Read the model definition and answer for the solid it produces. Units are mm, in the model's axes. Face numbers are marked on the shaded views. A direction names the side the tool comes from. Round coordinates to 2 decimals unless told otherwise and drop trailing zeros. Order: outer loops, then holes, each group sorted by start corner. A loop starts at its lowest first (then second) coordinate and runs counter-clockwise, first axis right, second up. Notation, with made-up numbers: (85, -8.75) - (107, -8.75) arc R16 ccw to (107, -1.75) - close; hole circle Ø2 at (38.25, -29.75). An arc over 180 degrees is marked (long way). Answer as a JSON object with one key per item and string values. Group by question number.
Q1. A cutting plane is placed at C-C on z = -47.75. Determine the outline of the cut face in (x, y) (3 decimals), and give its area (3 significant figures).
Q2. A tool of negligible diameter and unlimited length cuts with its end or side. For the marked faces 1 and 2, from which of +Z, -Z, +X, -X, +Y, -Y can it reach the whole face along a straight path? Write none if from no direction.
Q3. Given pin 1 Ø2 at (y, z) = (-19.5, -39) entering from +X; pin 2 Ø1 at (y, z) = (-30.5, -42.5) entering from +X; pin 3 Ø5 at (y, z) = (21.5, -49) entering from +X; pin 4 Ø1 at (x, y) = (6.5, -25) entering from +Z, each flat-ended and moving along its own axis, determine where each tip first touches the part or whether it passes through.
Q4. A cutting plane is placed at A-A on x = 12.5. Determine the outline of the cut face in (y, z) (3 decimals), and give its area (3 significant figures).
Q5. A cutting plane is placed at B-B on y = -30.1. Determine the outline of the cut face in (x, z) (3 decimals), and give its area (3 significant figures).
Q6. A cutting plane is placed at D-D on z = -1. Determine the outline of the cut face in (x, y).
Q7. Consider line 1 (Y direction, x = 3.7, z = -47.75) (3 decimals); line 2 (Y direction, x = 10.65, z = 45) (3 decimals); line 3 (Y direction, x = 1.2, z = -61.09). Determine where each line is inside the solid, lowest interval first.
```python
from build123d import *

# Parameters (mm, degrees)
SKETCH1_W            = 133.35
SKETCH1_H            = 76.2
BOSS_EXTRUDE1_DEPTH  = 5
FILLET1_R            = 3.175
SKETCH2_R            = 3.025
CUT_EXTRUDE1_DEPTH   = 77.955608145
SKETCH5_R            = 3.25
SKETCH5_R_2          = 1.665
BOSS_EXTRUDE2_DEPTH  = 2
CUT_EXTRUDE2_START   = -6
SKETCH6_R            = 1.665
CUT_EXTRUDE2_DEPTH   = 6
SKETCH8_R            = 3.75
BOSS_EXTRUDE4_DEPTH  = 9
SKETCH9_R            = 1.665
CUT_EXTRUDE3_DEPTH   = 5
M4_CLEARANCE_HOLE1_D = 4.8
SKETCH16_R           = 4.25
SKETCH16_R_2         = 2.4
CUT_EXTRUDE4_DEPTH   = 2.5


with BuildPart() as part:
    # Sketch1 → Boss-Extrude1 (new body)
    with BuildSketch(Plane(origin=(0, 0, 0), x_dir=(0, 0, -1), z_dir=(1, 0, 0))):
        Rectangle(SKETCH1_W, SKETCH1_H)
    extrude(amount=BOSS_EXTRUDE1_DEPTH)

    # Fillet1
    fillet1_edges = [part.edges().sort_by_distance(p)[0] for p in [
        (2.5, -38.1, -66.675),
        (2.5, -38.1, 66.675),
        (2.5, 38.1, 66.675),
        (2.5, 38.1, -66.675),
    ]]
    fillet(fillet1_edges, radius=FILLET1_R)

    # Sketch2 → Cut-Extrude1 (cut, through all)
    with BuildSketch(Plane.ZY):
        with Locations((-61.09, -22.225)):
            Circle(SKETCH2_R)
        with Locations((-61.09, 22.225)):
            Circle(SKETCH2_R)
        with Locations((61.09, -22.225)):
            Circle(SKETCH2_R)
        with Locations((61.09, 22.225)):
            Circle(SKETCH2_R)
    extrude(amount=-CUT_EXTRUDE1_DEPTH, mode=Mode.SUBTRACT)

    # Sketch5 → Boss-Extrude2 (add)
    # profile 1 of 4: a face of its own
    with BuildSketch(Plane(origin=(5, 0, 0), x_dir=(0, 0, -1), z_dir=(1, 0, 0))):
        with Locations((-52.75, 23)):
            Circle(SKETCH5_R)
        with Locations((-52.75, 23)):
            Circle(SKETCH5_R_2, mode=Mode.SUBTRACT)
    # profile 2 of 4: a face of its own
    with BuildSketch(Plane(origin=(5, 0, 0), x_dir=(0, 0, -1), z_dir=(1, 0, 0))):
        with Locations((-52.75, -12)):
            Circle(SKETCH5_R)
        with Locations((-52.75, -12)):
            Circle(SKETCH5_R_2, mode=Mode.SUBTRACT)
    # profile 3 of 4: a face of its own
    with BuildSketch(Plane(origin=(5, 0, 0), x_dir=(0, 0, -1), z_dir=(1, 0, 0))):
        with Locations((47.75, 23)):
            Circle(SKETCH5_R)
        with Locations((47.75, 23)):
            Circle(SKETCH5_R_2, mode=Mode.SUBTRACT)
    # profile 4 of 4: a face of its own
    with BuildSketch(Plane(origin=(5, 0, 0), x_dir=(0, 0, -1), z_dir=(1, 0, 0))):
        with Locations((47.75, -12)):
            Circle(SKETCH5_R)
    extrude(amount=BOSS_EXTRUDE2_DEPTH)

    # Sketch6 → Cut-Extrude2 (cut)
    with BuildSketch(Plane(origin=(7, 0, 0), x_dir=(0, 0, -1), z_dir=(1, 0, 0)).offset(CUT_EXTRUDE2_START)):
        with Locations((-52.75, -12)):
            Circle(SKETCH6_R)
        with Locations((-52.75, 23)):
            Circle(SKETCH6_R)
        with Locations((47.75, -12)):
            Circle(SKETCH6_R)
        with Locations((47.75, 23)):
            Circle(SKETCH6_R)
    extrude(amount=CUT_EXTRUDE2_DEPTH, mode=Mode.SUBTRACT)

    # Sketch8 → Boss-Extrude4 (add)
    with BuildSketch(Plane(origin=(5, 0, 0), x_dir=(0, 0, -1), z_dir=(1, 0, 0))):
        with Locations((-45, -30.1)):
            Circle(SKETCH8_R)
        with Locations((-45, 30.1)):
            Circle(SKETCH8_R)
        with Locations((42, 30.1)):
            Circle(SKETCH8_R)
        with Locations((42, -30.1)):
            Circle(SKETCH8_R)
    extrude(amount=BOSS_EXTRUDE4_DEPTH)

    # Sketch9 → Cut-Extrude3 (cut)
    with BuildSketch(Plane(origin=(14, 0, 0), x_dir=(0, 0, -1), z_dir=(1, 0, 0))):
        with Locations((-45, -30.1)):
            Circle(SKETCH9_R)
        with Locations((-45, 30.1)):
            Circle(SKETCH9_R)
        with Locations((42, 30.1)):
            Circle(SKETCH9_R)
        with Locations((42, -30.1)):
            Circle(SKETCH9_R)
    extrude(amount=-CUT_EXTRUDE3_DEPTH, mode=Mode.SUBTRACT)

    # M4 Clearance Hole1 (through all)
    with Locations(Plane(origin=(-0.0007, 0, 61.8815), x_dir=(0, 0, -1), z_dir=(-1, 0, 0))):
        with Locations((0, 0), (123.763, 0)):
            Hole(M4_CLEARANCE_HOLE1_D / 2)

    # Sketch16 → Cut-Extrude4 (cut)
    # profile 1 of 6: a face of its own
    with BuildSketch(Plane(origin=(5, 0, 0), x_dir=(0, 0, -1), z_dir=(1, 0, 0))):
        with Locations((-61.8815, 0)):
            Circle(SKETCH16_R)
        with Locations((-61.8815, 0)):
            Circle(SKETCH16_R_2, mode=Mode.SUBTRACT)
    # profile 2 of 6: a face of its own
    with BuildSketch(Plane(origin=(5, 0, 0), x_dir=(0, 0, -1), z_dir=(1, 0, 0))):
        with BuildLine():
            ThreePointArc((-61.8815, -4.25), (-66.1315, 0), (-61.8815, 4.25))
            Line((-61.8815, 4.25), (-66.675, 4.25))
            Line((-66.675, 4.25), (-66.675, -4.25))
            Line((-66.675, -4.25), (-61.8815, -4.25))
        make_face()
    # profile 3 of 6: a face of its own
    with BuildSketch(Plane(origin=(5, 0, 0), x_dir=(0, 0, -1), z_dir=(1, 0, 0))):
        with Locations((-61.8815, 0)):
            Circle(SKETCH16_R_2)
    # profile 4 of 6: a face of its own
    with BuildSketch(Plane(origin=(5, 0, 0), x_dir=(0, 0, -1), z_dir=(1, 0, 0))):
        with Locations((61.8815, 0)):
            Circle(SKETCH16_R)
        with Locations((61.8815, 0)):
            Circle(SKETCH16_R_2, mode=Mode.SUBTRACT)
    # profile 5 of 6: a face of its own
    with BuildSketch(Plane(origin=(5, 0, 0), x_dir=(0, 0, -1), z_dir=(1, 0, 0))):
        with BuildLine():
            Line((66.675, 4.25), (61.8815, 4.25))
            ThreePointArc((61.8815, 4.25), (64.88670382, 3.00520382), (66.1315, 0))
            ThreePointArc((66.1315, 0), (64.88670382, -3.00520382), (61.8815, -4.25))
            Line((61.8815, -4.25), (66.675, -4.25))
            Line((66.675, -4.25), (66.675, 4.25))
        make_face()
    # profile 6 of 6: a face of its own
    with BuildSketch(Plane(origin=(5, 0, 0), x_dir=(0, 0, -1), z_dir=(1, 0, 0))):
        with Locations((61.8815, 0)):
            Circle(SKETCH16_R_2)
    extrude(amount=-CUT_EXTRUDE4_DEPTH, mode=Mode.SUBTRACT)


solid = part.part
```
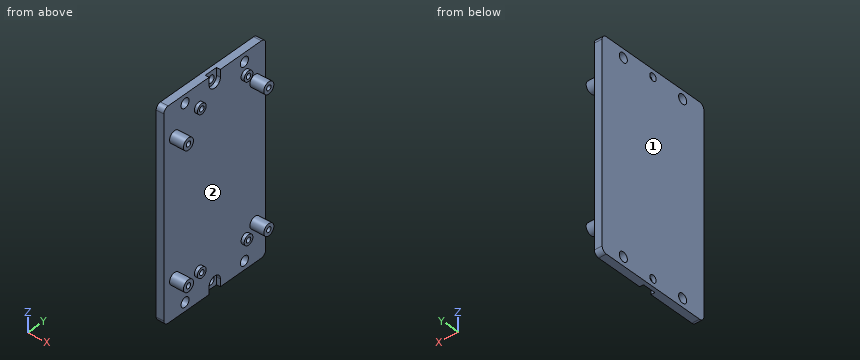
Result set:
{
 "1": {"outline": "(0, -38.1) - (5, -38.1) - (5, -15.25) - (7, -15.25) - (7, -13.665) - (1, -13.665) - (1, -10.335) - (7, -10.335) - (7, -8.75) - (5, -8.75) - (5, 19.75) - (7, 19.75) - (7, 21.335) - (1, 21.335) - (1, 24.665) - (7, 24.665) - (7, 26.25) - (5, 26.25) - (5, 38.1) - (0, 38.1) - close", "area": "367 mm²"},
 "2": {"face 1": "+Z, -Z, -X, +Y, -Y", "face 2": "+X"},
 "3": {"pin 1": "stops at x = 5", "pin 2": "stops at x = 9", "pin 3": "stops at x = 7", "pin 4": "passes through"},
 "4": {"outline": "circle Ø7.5 at (-30.1, -42); circle Ø7.5 at (-30.1, 45); circle Ø7.5 at (30.1, -42); circle Ø7.5 at (30.1, 45); hole circle Ø3.33 at (-30.1, -42); hole circle Ø3.33 at (-30.1, 45); hole circle Ø3.33 at (30.1, -42); hole circle Ø3.33 at (30.1, 45)", "area": "142 mm²"},
 "5": {"outline": "(0, -66.675) - (5, -66.675) - (5, -45.75) - (14, -45.75) - (14, -43.665) - (9, -43.665) - (9, -40.335) - (14, -40.335) - (14, -38.25) - (5, -38.25) - (5, 41.25) - (14, 41.25) - (14, 43.335) - (9, 43.335) - (9, 46.665) - (14, 46.665) - (14, 48.75) - (5, 48.75) - (5, 66.675) - (0, 66.675) - close", "area": "768 mm²"},
 "6": {"outline": "(0, -38.1) - (5, -38.1) - (5, 38.1) - (0, 38.1) - close"},
 "7": {"line 1": "y = -38.1 to -13.665, -10.335 to 21.335, 24.665 to 38.1", "line 2": "y = -33.85 to -31.765, -28.435 to -26.35, 26.35 to 28.435, 31.765 to 33.85", "line 3": "y = -38.1 to -25.25, -19.2 to -2.27, 2.27 to 19.2, 25.25 to 38.1"}
}
